from build123d import *
from build123d.topology import SkipClean

# Parameters (mm, degrees)
SKETCH_1_R          = 13
SKETCH_1_R_2        = 4
EXTRUDE_1_DEPTH     = 15
EXTRUDE_1_2_DEPTH   = 15
EXTRUDE_2_DEPTH     = 4.5
CUT_EXTRUDE_1_DEPTH = 2


with BuildPart() as part:
    # Sketch 1 → Extrude 1 (new, symmetric)
    with BuildSketch(Plane(origin=(0, 0, 0), x_dir=(1, 0, 0), z_dir=(0, 1, 0))):
        with Locations(Location((-118, 0, 0), (0, 0, 270))):
            Circle(SKETCH_1_R)
        with Locations(Location((-118, 0, 0), (0, 0, 270))):
            Circle(SKETCH_1_R_2, mode=Mode.SUBTRACT)
    extrude(amount=EXTRUDE_1_DEPTH, both=True)



with BuildPart() as body_2:
    # Sketch 1 → Extrude 1 2 (new, symmetric)
    with BuildSketch(Plane(origin=(0, 0, 0), x_dir=(1, 0, 0), z_dir=(0, 1, 0))):
        with Locations(Location((-13, 0, 0), (0, 0, 270))):
            Circle(SKETCH_1_R)
        with Locations(Location((-13, 0, 0), (0, 0, 270))):
            Circle(SKETCH_1_R_2, mode=Mode.SUBTRACT)
    extrude(amount=EXTRUDE_1_2_DEPTH, both=True)


with BuildPart() as part_1:
    add(part.part)

    add(body_2.part)  # Extrude 2 merges body 2
    # Sketch 2 → Extrude 2 (add, symmetric)
    with BuildSketch(Plane(origin=(0, 0, 0), x_dir=(1, 0, 0), z_dir=(0, 1, 0))):
        with BuildLine():
            Line((-111.07179677, 11), (-19.92820323, 11))
            ThreePointArc((-19.92820323, 11), (-26, 0), (-19.92820323, -11))
            Line((-19.92820323, -11), (-111.07179677, -11))
            ThreePointArc((-111.07179677, -11), (-105, 0), (-111.07179677, 11))
        make_face()
    extrude(amount=EXTRUDE_2_DEPTH, both=True)

    # Sketch 4 → Cut-Extrude 1 (cut)
    with SkipClean():  # the faces are left unmerged after this step: merging them gives an invalid solid
        with BuildSketch(Plane(origin=(0, 4.5, 0), x_dir=(1, 0, 0), z_dir=(0, 1, 0))):
            with BuildLine():
                Line((-106.467437405, 6), (-24.532562595, 6))
                ThreePointArc((-24.532562595, 6), (-26, 0), (-24.532562595, -6))
                Line((-24.532562595, -6), (-106.467437405, -6))
                ThreePointArc((-106.467437405, -6), (-105, 0), (-106.467437405, 6))
            make_face()
        cut_extrude_1 = extrude(amount=-CUT_EXTRUDE_1_DEPTH, mode=Mode.SUBTRACT)

    # Mirror 1: Cut-Extrude 1 across plane
    add(cut_extrude_1.mirror(Plane.ZX), mode=Mode.SUBTRACT)


solid = part_1.part
Geometry: final body of the model. Coordinates: model frame, mm. A direction names the side the tool comes from. Give positions to 0.01 mm unless a question says otherwise; leave off trailing zeros. Write each loop counter-clockwise with the first axis right and the second up, starting at its lowest first coordinate (ties: lowest second). Pieces come first, ordered by that corner, then holes. Notation, with made-up numbers: M -29,-19 L 25,-19 A22 cw 25,-8 Z; hole C -2,15.5 d5. An arc over 180 degrees is marked long. Answer in a Markdown table with one row per item. Add a question column.
(1) First-contact query: pin 1 (1.6 mm diameter, centred on x = -76.5, y = 3.5, fed in from +Z); pin 2 (8 mm diameter, centred on x = -87, y = -6.5, fed in from -Z); pin 3 (8 mm diameter, centred on x = -68, z = 3.5, fed in from +Y). Flat tips, straight axial feed; report the tip coordinate or a pass-through.
(2) Section D-D on x = -53.5. Return loops of the section in (y, z), and give its area (3 significant figures).
(3) Section C-C on y = -12.5. Return loops of the section in (x, z), and give its area (3 significant figures).
(4) Section B-B on z = 0. Return loops of the section in (x, y).
(5) Mould query, pull axis X, two halves, no side actions, for faces 4 (the flat face through (-65, 2.5, 0)), 5 (the cylindrical face through (-114.034, -0.21, -0.521)), 6 (the flat face through (-115, -15, 3)). Classes: +X half, -X half, draft (parallel to the pull), parting line (faces both ways), or undercut.
(6) Reachability of faces 1 (the flat face through (-65, 4.5, 8)), 2 (the flat face through (-66, 0, -11)), 3 (the flat face through (-65, 0, 11)) from +Z, -Z, +X, -X, +Y, -Y: full face, straight path, thin tool, end or side. Return the list, or none.
(7) Section A-A on x = -118. Return loops of the section in (y, z), and give its area (3 significant figures).
(8) Ray query, line 1 (X direction, y = -9, z = 0); line 2 (X direction, y = 1, z = 0); line 3 (X direction, y = 6, z = -0.75). Return the intervals inside material, ascending.
Result set:
| question | item | result |
|---|---|---|
| 1 | pin 1 | stops at z = 11 |
| 1 | pin 2 | stops at z = -11 |
| 1 | pin 3 | stops at y = 4.5 |
| 2 | outline | M -4.5,-11 L 4.5,-11 L 4.5,-6 L 2.5,-6 L 2.5,6 L 4.5,6 L 4.5,11 L -4.5,11 L -4.5,6 L -2.5,6 L -2.5,-6 L -4.5,-6 Z |
| 2 | area | 150 mm^2 |
| 3 | outline | C -118,0 d26; C -13,0 d26; hole C -118,0 d8; hole C -13,0 d8 |
| 3 | area | 961 mm^2 |
| 4 | outline | M -131,-15 L -122,-15 L -122,15 L -131,15 Z; M -114,-15 L -105,-15 L -105,-2.5 L -26,-2.5 L -26,-15 L -17,-15 L -17,15 L -26,15 L -26,2.5 L -105,2.5 L -105,15 L -114,15 Z; M -9,-15 L 0,-15 L 0,15 L -9,15 Z |
| 5 | face 4 | undercut |
| 5 | face 5 | undercut |
| 5 | face 6 | draft |
| 6 | face 1 | +Z, +Y |
| 6 | face 2 | -Z, +Y, -Y |
| 6 | face 3 | +Z, +Y, -Y |
| 7 | outline | M -15,-13 L 15,-13 L 15,-4 L -15,-4 Z; M -15,4 L 15,4 L 15,13 L -15,13 Z |
| 7 | area | 540 mm^2 |
| 8 | line 1 | x = -131 to -122, -114 to -105, -26 to -17, -9 to 0 |
| 8 | line 2 | x = -131 to -122, -114 to -17, -9 to 0 |
| 8 | line 3 | x = -130.98 to -121.93, -114.07 to -105.02, -25.98 to -16.93, -9.07 to -0.02 |
